```python
from build123d import *

# Parameters (mm, degrees)
F0_R     = 26.035
F0_R_2   = 12.5
F1_DEPTH = 15
F2_R     = 22.074638
F2_R_2   = 16.838659
F3_DEPTH = 1.5
F4_R     = 21.491301
F4_R_2   = 16.261001
F5_DEPTH = 1.5
F6_SIZE  = 1


with BuildPart() as f1:
    # F0 (on Front) → F1 (new body)
    with BuildSketch(Plane.XZ):
        Circle(F0_R)
        Circle(F0_R_2, mode=Mode.SUBTRACT)
    extrude(amount=F1_DEPTH)

    # F2 (on face) → F3 (cut)
    with BuildSketch(Plane.XZ.offset(15)):
        Circle(F2_R)
        Circle(F2_R_2, mode=Mode.SUBTRACT)
    extrude(amount=-F3_DEPTH, mode=Mode.SUBTRACT)

    # F4 (on face) → F5 (cut)
    with BuildSketch(Plane(origin=(0, 0, 0), x_dir=(-1, 0, 0), z_dir=(0, 1, 0))):
        Circle(F4_R)
        Circle(F4_R_2, mode=Mode.SUBTRACT)
    extrude(amount=-F5_DEPTH, mode=Mode.SUBTRACT)

    # F6
    f6_edges = [f1.edges().sort_by_distance(p)[0] for p in [
        (-26.035, 0, 0),
        (-26.035, -15, 0),
        (-12.5, -15, 0),
        (-12.5, 0, 0),
    ]]
    chamfer(f6_edges, length=F6_SIZE)


solid = f1.part
```
Could you check a few things on this model? Use its own coordinates, in mm. A direction names the side the tool comes from. Round coordinates to 2 decimals unless told otherwise and drop trailing zeros. Loops run counter-clockwise (first coordinate to the right, second up) from the corner with the lowest first, then second, coordinate; pieces in that order, holes last. Notation, with made-up numbers: (79.25, -22) -> (103.25, -22) arc R17 cw to (103.25, -16) -> close; hole circle Ø8 at (28, 5.5). An arc over 180 degrees is marked (long way). Put each result on its own line as item: value.
Q1. I want a section at C-C on y = -6.75. Write out the boundary of the cut face in (x, z) (3 decimals), and give its area (3 significant figures).
Checks:
outline: circle Ø52.07 at (0, 0); hole circle Ø25 at (0, 0)
area: 1,640 mm2
Q2. For pin 1 Ø6 at (x, y) = (-13, -10.5) entering from -Z; pin 2 Ø8 at (x, y) = (19.5, -2.5) entering from -Z; pin 3 Ø8 at (x, y) = (-2.5, -4.5) entering from +Z (3 decimals), each with a flat end and sliding along its axis, tell me the tip position at first contact or that it passes through.
Checks:
pin 1: z = -24.04
pin 2: z = -20.92
pin 3: z = 26.035
Q3. Please list where these lines run through material, in increasing order: line 1 (Z direction, x = 9, y = -14.25); line 2 (Z direction, x = 0, y = -0.5) (3 decimals); line 3 (X direction, y = -1, z = 7). Write a range as from..to.
Checks:
line 1: -24.16..-20.16, -14.23..-9.03, 9.03..14.23, 20.16..24.16
line 2: -25.535..-21.491, -16.261..-13, 13..16.261, 21.491..25.535
line 3: -25.08..-20.32, -14.68..-10.36, 10.36..14.68, 20.32..25.08
Q4. Thinking about a two-plate mould opening in Z: for faces 1 (the flat face through (15, -15, -17)), 2 (the cylindrical face through (16.06, -14.26, 5.06)), 3 (the flat face through (-5.01, -13.5, -16.25)), 4 (the cylindrical face through (-3.389, -7.409, 25.813)), which applies, pulls with the +Z half, pulls with the -Z half, needs draft (parallel to the pull), parting line crosses it, or undercut?
Checks:
face 1: needs draft
face 2: undercut
face 3: undercut
face 4: parting line crosses it
Q5. Which directions (+Z, -Z, +X, -X, +Y, -Y) give clear straight access to the entire face, cutting with the end or side of a thin tool? Please do faces 5 (the flat face through (-13, -15, 5)), 6 (the cylindrical face through (-15.51, -0.74, 4.88)), 7 (the cylindrical face through (-22.053, -14.26, 0.971)).
Checks:
face 5: +Z, -Z, +X, -X, -Y
face 6: +Y
face 7: -Y
